Could you check a few things on this model? Use its own coordinates, in mm. A direction names the side the tool comes from. Round coordinates to 2 decimals unless told otherwise and drop trailing zeros. Order: outer loops, then holes, each group sorted by start corner. A loop starts at its lowest first (then second) coordinate and runs counter-clockwise, first axis right, second up. Notation, with made-up numbers: (36, 59.5) -> (81, 59.5) arc R22 ccw to (81, 70.5) -> close; hole circle Ø5 at (66.5, 56). An arc over 180 degrees is marked (long way). One line per question, with ' | ' between items.
```python
from build123d import *

# Parameters (mm, degrees)
SKETCH2_W               = 31.75
SKETCH2_H               = 6.35
SKETCH2_R               = 1.5875
BOSS_EXTRUDE1_DEPTH     = 2.54
SKETCH3_W               = 1.5875
SKETCH3_H               = 6.35
BOSS_EXTRUDE2_DEPTH     = 6.35
CUT_EXTRUDE1_DEPTH      = 20.850733771
CUT_EXTRUDE1_DEPTH_BACK = 20.850733771
SKETCH4_R               = 1.5875
FILLET1_R               = 3.175


with BuildPart() as part:
    # Sketch2 → Boss-Extrude1 (new body)
    with BuildSketch(Plane(origin=(0, 0, 0), x_dir=(1, 0, 0), z_dir=(0, 1, 0))):
        Rectangle(SKETCH2_W, SKETCH2_H)
        with Locations(Location((-12.7, 0, 0), (0, 0, 270))):
            Circle(SKETCH2_R, mode=Mode.SUBTRACT)
        with Locations(Location((12.7, 0, 0), (0, 0, 270))):
            Circle(SKETCH2_R, mode=Mode.SUBTRACT)
    extrude(amount=BOSS_EXTRUDE1_DEPTH)

    # Sketch3 → Boss-Extrude2 (add)
    with BuildSketch(Plane(origin=(0, 2.54, 0), x_dir=(1, 0, 0), z_dir=(0, 1, 0))):
        with Locations((-2.38125, 0)):
            Rectangle(SKETCH3_W, SKETCH3_H)
        with Locations((2.38125, 0)):
            Rectangle(SKETCH3_W, SKETCH3_H)
    extrude(amount=BOSS_EXTRUDE2_DEPTH)

    # Sketch4 → Cut-Extrude1 (cut, two sides: drawn at the far end of the back side and taken through both)
    with BuildSketch(Plane(origin=(-1.5875, 0, 0), x_dir=(0, 0, -1), z_dir=(1, 0, 0)).offset(-CUT_EXTRUDE1_DEPTH_BACK)):
        with Locations((0, 5.715)):
            Circle(SKETCH4_R)
    extrude(amount=CUT_EXTRUDE1_DEPTH + CUT_EXTRUDE1_DEPTH_BACK, mode=Mode.SUBTRACT)

    # Fillet1
    fillet1_edges = [part.edges().sort_by_distance(p)[0] for p in [
        (-15.875, 1.27, 3.175),
        (-15.875, 1.27, -3.175),
        (15.875, 1.27, -3.175),
        (15.875, 1.27, 3.175),
        (2.38125, 8.89, 3.175),
        (2.38125, 8.89, -3.175),
        (-2.38125, 8.89, -3.175),
        (-2.38125, 8.89, 3.175),
    ]]
    fillet(fillet1_edges, radius=FILLET1_R - 0.0001)  # a hair under: the kernel refuses the full size


solid = part.part
```
1. On a 3-axis mill with a long thin cutter (end or side, diameter ignored), from which of +Z, -Z, +X, -X, +Y, -Y can I reach the whole of each face in a straight line? I mean faces 1 (the face through (0, 2, 3.175)), 2 (the face through (9, 2.54, 0)), 3 (the face through (0, 2.54, 0)), 4 (the face through (-8, 2.54, 0)). Say none if no direction works.
From the geometry:
face 1: +Z, +X, -X, +Y, -Y | face 2: +Z, -Z, +X, +Y | face 3: +Z, -Z, +Y | face 4: +Z, -Z, -X, +Y
2. I want a section at A-A on y = 3.5. List the corners of the cut face in (x, z) for me (1 decimal).
From the geometry:
outline: (-3.2, -3.2) -> (-1.6, -3.2) -> (-1.6, 3.2) -> (-3.2, 3.2) -> close; (1.6, -3.2) -> (3.2, -3.2) -> (3.2, 3.2) -> (1.6, 3.2) -> close
3. I'm going to push flat-ended pins straight in: pin 1 (3 mm diameter, centred on x = -12.7, z = 0, fed in from +Y); pin 2 (3 mm diameter, centred on x = 8.5, z = -0.5, fed in from +Y); pin 3 (1.9 mm diameter, centred on y = 7, z = 0, fed in from +X) (3 decimals). Where does each tip first touch, or does it pass through?
From the geometry:
pin 1: passes through | pin 2: stops at y = 2.54 | pin 3: stops at x = 3.175
4. If we mould it in two halves opening along Z, with no side actions, what happens to faces 5 (the face through (-2.37, 7.935, -2.27)), 6 (the face through (-3.175, 4, -1)), 7 (the face through (2.37, 7.29, 0.21)), 8 (the face through (-11.126, 1.252, -0.207))? For each: pulls with the +Z half, pulls with the -Z half, needs draft (parallel to the pull), parting line crosses it, or undercut.
From the geometry:
face 5: pulls with the -Z half | face 6: needs draft | face 7: undercut | face 8: undercut
5. I want a section at C-C on z = -0.75. List the corners of the cut face in (x, y) for me (1 decimal), and give its area (3 significant figures).
From the geometry:
outline: (-15.8, 0) -> (-14.1, 0) -> (-14.1, 2.5) -> (-15.8, 2.5) -> close; (-11.3, 0) -> (11.3, 0) -> (11.3, 2.5) -> (3.2, 2.5) -> (3.2, 4.3) -> (1.6, 4.3) -> (1.6, 2.5) -> (-1.6, 2.5) -> (-1.6, 4.3) -> (-3.2, 4.3) -> (-3.2, 2.5) -> (-11.3, 2.5) -> close; (-3.2, 7.1) -> (-1.6, 7.1) -> (-1.6, 8.8) -> (-3.2, 8.8) -> close; (1.6, 7.1) -> (3.2, 7.1) -> (3.2, 8.8) -> (1.6, 8.8) -> close; (14.1, 0) -> (15.8, 0) -> (15.8, 2.5) -> (14.1, 2.5) -> close | area: 77.0 mm²
6. I want a section at D-D on z = 2.5. List the corners of the cut face in (x, y) for me (1 decimal).
From the geometry:
outline: (-14.7, 0) -> (14.7, 0) -> (14.7, 2.5) -> (3.2, 2.5) -> (3.2, 7.7) -> (1.6, 7.7) -> (1.6, 2.5) -> (-1.6, 2.5) -> (-1.6, 7.7) -> (-3.2, 7.7) -> (-3.2, 2.5) -> (-14.7, 2.5) -> close
7. I want a section at B-B on y = 2. Count the separate pieces of the cut face and the enclosed holes in it, and give its area (3 significant figures).
From the geometry:
separate pieces: 1 | enclosed holes: 2 | area: 177 mm²
8. I need wall thicknesses on probe 1 along X at (y, z) = (1.2, 0) (1 decimal); probe 2 along X at (y, z) = (6, 2.5) (1 decimal); probe 3 along Y at (x, z) = (2.25, 0). Which ranges of each line are inside material? Lowest first, please.
From the geometry:
probe 1: x = -15.9 to -14.3, -11.1 to 11.1, 14.3 to 15.9 | probe 2: x = -3.2 to -1.6, 1.6 to 3.2 | probe 3: y = 0 to 4.13, 7.3 to 8.89
